Source: three-view drawing plus pictorial views. Frame: mm from the lowest corner of the part. A direction names the side the tool comes from. Round coordinates to 2 decimals unless told otherwise and drop trailing zeros. Order: outer loops, then holes, each group sorted by start corner. A loop starts at its lowest first (then second) coordinate and runs counter-clockwise, first axis right, second up. Notation, with made-up numbers: M 83.25,57.5 L 123.25,57.5 A32 ccw 123.25,95.5 Z; hole C -19,-15.75 d10. An arc over 180 degrees is marked long. Return JSON: item names as keys, results as strings. Group by question number.
Q1. Mould query, pull axis Y, two halves, no side actions, for the marked faces 1, 2 and 3. Classes: released by +Y, released by -Y, zero draft, split by the parting line, or undercut.
Q2. Cut plane B-B on y = 41. Output: boundary loops of the cut face in (x, z).
Q3. Cut plane D-D on y = 12. Output: boundary loops of the cut face in (x, z), and give its area (3 significant figures).
Q4. Access query for the marked faces 4, 5 and 6. Directions: +Z, -Z, +X, -X, +Y, -Y. A direction counts if a zero-diameter tool reaches every point of the face in a straight line with its end or side. Return the directions, or none.
Q5. Ray query, probe 1 along Y at (x, z) = (5, 41); probe 2 along X at (y, z) = (4, 16); probe 3 along Z at (x, y) = (33.5, 35.5). Return the intervals inside material, ascending.
Q6. Cut plane A-A on z = 28.5. Output: boundary loops of the cut face in (x, y).
Q7. Cut plane C-C on x = 77. Output: boundary loops of the cut face in (y, z).
Q8. Contact query for a flat-ended pin moving along its axis: pin 1 (10 mm diameter, centred on x = 29.5, y = 24, fed in from -Z). Output: stop coordinate, or through.
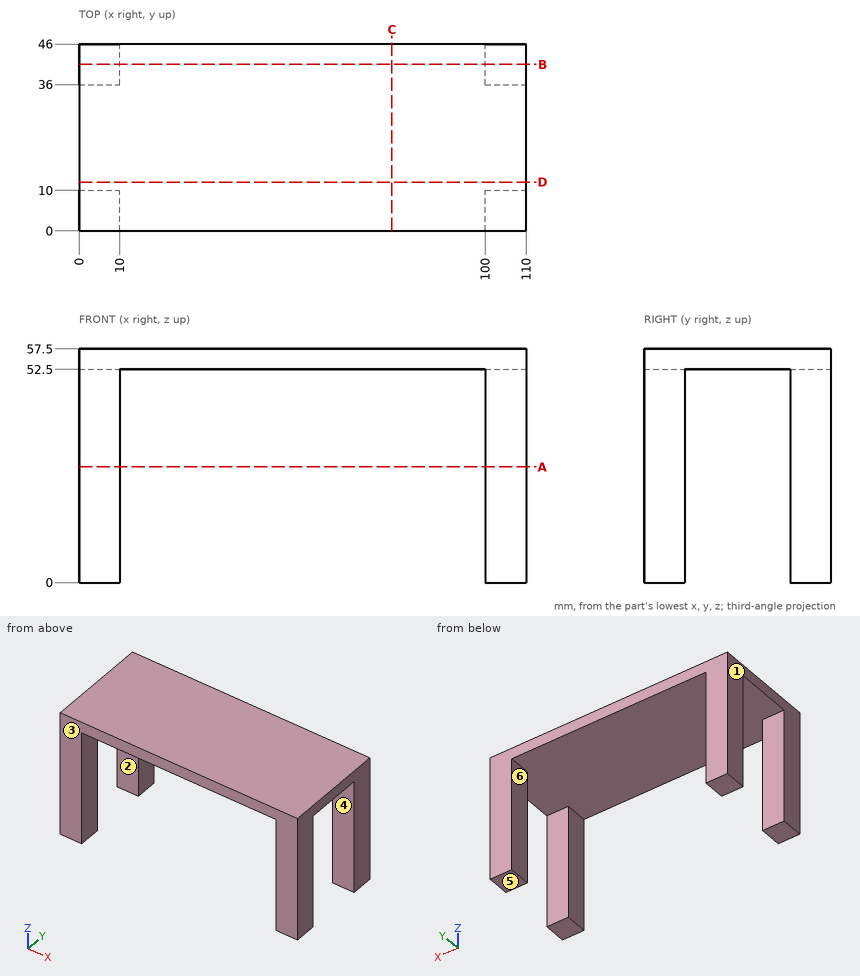
Result sheet:
{
 "1": {"face 1": "zero draft", "face 2": "undercut", "face 3": "released by -Y"},
 "2": {"outline": "M 0,0 L 10,0 L 10,52.5 L 100,52.5 L 100,0 L 110,0 L 110,57.5 L 0,57.5 Z"},
 "3": {"outline": "M 0,52.5 L 110,52.5 L 110,57.5 L 0,57.5 Z", "area": "550 mm²"},
 "4": {"face 4": "-Z, +X, -X", "face 5": "-Z, +X, -X, +Y, -Y", "face 6": "-Z, +Y, -Y"},
 "5": {"probe 1": "y = 0 to 10, 36 to 46", "probe 2": "x = 0 to 10, 100 to 110", "probe 3": "z = 52.5 to 57.5"},
 "6": {"outline": "M 0,0 L 10,0 L 10,10 L 0,10 Z; M 0,36 L 10,36 L 10,46 L 0,46 Z; M 100,0 L 110,0 L 110,10 L 100,10 Z; M 100,36 L 110,36 L 110,46 L 100,46 Z"},
 "7": {"outline": "M 0,52.5 L 46,52.5 L 46,57.5 L 0,57.5 Z"},
 "8": {"pin 1": "stops at z = 52.5"}
}
